Could you check a few things on this model? Use its own coordinates, in mm. A direction names the side the tool comes from. Give positions to 0.01 mm unless a question says otherwise; leave off trailing zeros. Loops run counter-clockwise (first coordinate to the right, second up) from the corner with the lowest first, then second, coordinate; pieces in that order, holes last. Notation, with made-up numbers: (59.5, -27.75) - (72.5, -27.75) arc R16 ccw to (72.5, -23.75) - close; hole circle Ø5 at (23, 1.25). An arc over 180 degrees is marked (long way). One line per item, written item: value. Start each with the question number.
Q1. I want a section at A-A (x = -7.5). Please give me the cut outline in (y, z), then the cut area to 3 significant figures.
Q2. I want a section at C-C (y = 10.75). Count the separate pieces of the cut face and the enclosed holes in it, then the cut area to 3 significant figures.
Q3. I'm going to push a flat-ended pin straight in: P1, Ø3, axis at y = 20, z = 2.5, coming from the +X side. Where does the tip first touch, or does it pass through?
Q4. I want a section at B-B (y = 3.5). Please give me the cut outline in (x, z).
Q5. For faces 1 (the face through (7.91, 11.85, 5.38)), 2 (the face through (0, 23, 8)), 3 (the face through (9.699, 22.715, -2.536)), 4 (the face through (2.4, 18.5, 4.9)), which set-ups out of +Z, -Z, +X, -X, +Y, -Y let a thin tool reach every point of the face, with its end or its side?
Q6. If I drill on line 1 (X direction, y = 0.3, z = 2); line 2 (X direction, y = 5.25, z = 7.25); line 3 (Z direction, x = 1.75, y = 11.5), over which ranges is the centre line in solid material (lowest first)? Write a range as from..to.
Q7. If we mould it in two halves opening along X, with no side actions, what happens to faces 5 (the face through (10, 11, 7)), 6 (the face through (-9.54, 12.15, -1.19)), 7 (the face through (-9.715, 9.614, -7.199))? For each: released by +X, released by -X, zero draft, split by the parting line, or undercut.
```python
from build123d import *

# Parameters (mm, degrees)
SKETCH1_W           = 20
SKETCH1_H           = 24
SKETCH1_R           = 2
BOSS_EXTRUDE2_DEPTH = 1
BOSS_EXTRUDE3_DEPTH = 23
SKETCH1_5_R         = 2
BOSS_EXTRUDE4_DEPTH = 5
CUT_EXTRUDE1_DEPTH  = 23.5
FILLET2_R           = 3.5
FILLET1_R           = 1
CUT_EXTRUDE3_START  = -19.5
CUT_EXTRUDE3_DEPTH  = 18.5


with BuildPart() as part:
    # Sketch1 → Boss-Extrude2 (new body)
    with BuildSketch(Plane(origin=(0, 0, 0), x_dir=(1, 0, 0), z_dir=(0, 1, 0))):
        with Locations((0, -4.5)):
            Rectangle(SKETCH1_W, SKETCH1_H)
        with Locations(Location((-7, -2, 0), (0, 0, 270))):
            Circle(SKETCH1_R, mode=Mode.SUBTRACT)
        with Locations(Location((7, -2, 0), (0, 0, 270))):
            Circle(SKETCH1_R, mode=Mode.SUBTRACT)
    extrude(amount=BOSS_EXTRUDE2_DEPTH)

    # Sketch1<4> → Boss-Extrude3 (add)
    with BuildSketch(Plane(origin=(0, 0, 0), x_dir=(1, 0, 0), z_dir=(0, 1, 0))):
        with BuildLine():
            Line((10, 7.5), (-10, 7.5))
            Line((-10, 7.5), (-10, -0.197224362))
            ThreePointArc((-10, -0.197224362), (-6.064585653, 1.372684391), (-3.5, -2))
            ThreePointArc((-3.5, -2), (-6.064585653, -5.372684391), (-10, -3.802775638))
            Line((-10, -3.802775638), (-10, -16.5))
            Line((-10, -16.5), (10, -16.5))
            Line((10, -16.5), (10, -3.802775638))
            ThreePointArc((10, -3.802775638), (3.5, -2), (10, -0.197224362))
            Line((10, -0.197224362), (10, 7.5))
        make_face()
    extrude(amount=BOSS_EXTRUDE3_DEPTH)

    # Sketch2 → Cut-Extrude1 (cut)
    with BuildSketch(Plane.XY.offset(16.5)):
        with BuildLine():
            Line((-4.949747468, 15.949747468), (0, 20.899494937))
            Line((0, 20.899494937), (4.949747468, 15.949747468))
            ThreePointArc((4.949747468, 15.949747468), (0, 4), (-4.949747468, 15.949747468))
        make_face()
    extrude(amount=-CUT_EXTRUDE1_DEPTH, mode=Mode.SUBTRACT)

    # Fillet2
    fillet2_edges = [part.edges().sort_by_distance(p)[0] for p in [
        (0, 23, -7.5),
    ]]
    fillet(fillet2_edges, radius=FILLET2_R)

    # Fillet1
    fillet1_edges = [part.edges().sort_by_distance(p)[0] for p in [
        (10, 12, 3.802775638),
        (10, 12, 0.197224362),
        (-10, 12, 3.802775638),
        (-10, 12, 0.197224362),
        (-10, 11.5, 16.5),
        (10, 11.5, 16.5),
        (10, 9.75, -7.5),
        (-10, 9.75, -7.5),
        (10, 23, -1.901387819),
        (10, 21.974873734, -6.474873734),
        (-10, 23, -1.901387819),
        (-10, 21.974873734, -6.474873734),
    ]]
    fillet(fillet1_edges, radius=FILLET1_R)

    # Sketch4 → Cut-Extrude3 (cut)
    with BuildSketch(Plane.XZ.offset(CUT_EXTRUDE3_START)):
        with BuildLine():
            Line((-9.5, -2.251571667), (-9.5, -6))
            ThreePointArc((-9.5, -6), (-9.207106781, -6.707106781), (-8.5, -7))
            Line((-8.5, -7), (8.5, -7))
            ThreePointArc((8.5, -7), (9.207106781, -6.707106781), (9.5, -6))
            Line((9.5, -6), (9.5, -2))
            Line((9.5, -2), (9.4, -2))
            Line((9.4, -2), (9.4, -6))
            ThreePointArc((9.4, -6), (9.136396103, -6.636396103), (8.5, -6.9))
            Line((8.5, -6.9), (-8.5, -6.9))
            ThreePointArc((-8.5, -6.9), (-9.136396103, -6.636396103), (-9.4, -6))
            Line((-9.4, -6), (-9.4, -2.251571667))
            Line((-9.4, -2.251571667), (-9.5, -2.251571667))
        make_face()
    extrude(amount=CUT_EXTRUDE3_DEPTH, mode=Mode.SUBTRACT)


with BuildPart() as body_2:
    # Sketch1<5> → Boss-Extrude4 (new body)
    # profile 1 of 2: a face of its own
    with BuildSketch(Plane(origin=(0, 0, 0), x_dir=(1, 0, 0), z_dir=(0, 1, 0))):
        with BuildLine():
            ThreePointArc((-3.5, -2), (-6.064585653, 1.372684391), (-10, -0.197224362))
            Line((-10, -0.197224362), (-10, -3.802775638))
            ThreePointArc((-10, -3.802775638), (-6.064585653, -5.372684391), (-3.5, -2))
        make_face()
        with Locations(Location((-7, -2, 0), (0, 0, 270))):
            Circle(SKETCH1_5_R, mode=Mode.SUBTRACT)
    # profile 2 of 2: a face of its own
    with BuildSketch(Plane(origin=(0, 0, 0), x_dir=(1, 0, 0), z_dir=(0, 1, 0))):
        with Locations(Location((-7, -2, 0), (0, 0, 270))):
            Circle(SKETCH1_5_R)
    extrude(amount=BOSS_EXTRUDE4_DEPTH)


solid = part.part
```
Worked answers:
1. outline: (0, -7.5) - (19.5, -7.5) arc R3.5 ccw to (23, -4) - (23, -1.46) - (1, -1.46) - (1, 0.06) - (0, 0.06) - close; (0, 3.94) - (1, 3.94) - (1, 5.46) - (23, 5.46) - (23, 16.5) - (0, 16.5) - close; hole (1, -7) - (19.5, -7) - (19.5, -6.9) - (1, -6.9) - close
1. area: 391 mm²
2. separate pieces: 3
2. enclosed holes: 0
2. area: 109 mm²
3. P1: stops at x = 4.13
4. outline: (-10, -6.5) arc R1 ccw to (-9, -7.5) - (9, -7.5) arc R1 ccw to (10, -6.5) - (10, -2.03) arc R1 ccw to (8.56, -1.14) arc R3.5 cw (long way) to (8.56, 5.14) arc R1 ccw to (10, 6.03) - (10, 15.5) arc R1 ccw to (9, 16.5) - (-9, 16.5) arc R1 ccw to (-10, 15.5) - (-10, 6.03) arc R1 ccw to (-8.56, 5.14) arc R3.5 cw (long way) to (-8.56, -1.14) arc R1 ccw to (-10, -2.03) - close; hole (-9.5, -6) arc R1 ccw to (-8.5, -7) - (8.5, -7) arc R1 ccw to (9.5, -6) - (9.5, -2) - (9.4, -2) - (9.4, -6) arc R0.9 cw to (8.5, -6.9) - (-8.5, -6.9) arc R0.9 cw to (-9.4, -6) - (-9.4, -2.25) - (-9.5, -2.25) - close
5. face 1: +Y
5. face 2: +Z, -Z, +X, -X, +Y
5. face 3: -Z, +X, +Y
5. face 4: +Z
6. line 1: x = -10..-9, -5..5, 9..10
6. line 2: x = -10..-3.99, 3.99..10
6. line 3: z = -7.5..-7
7. face 5: released by +X
7. face 6: undercut
7. face 7: released by -X
